For this review, take the finished solid that the model builds, in its own axes (mm). Face numbers are marked on the shaded views. A direction names the side the tool comes from. Round coordinates to 2 decimals unless told otherwise and drop trailing zeros. Order: outer loops, then holes, each group sorted by start corner. A loop starts at its lowest first (then second) coordinate and runs counter-clockwise, first axis right, second up.
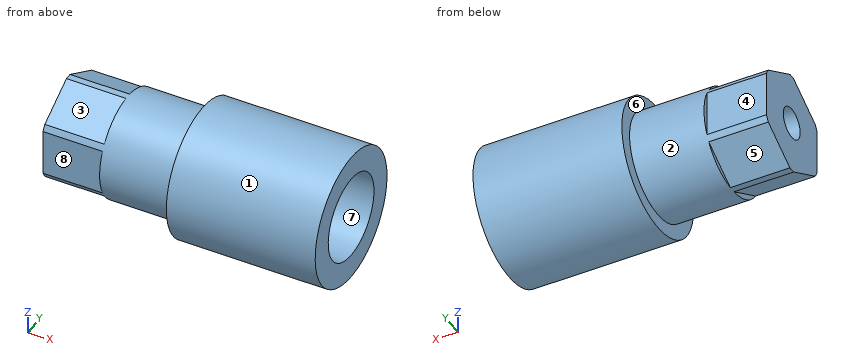
from build123d import *

# Parameters (mm, degrees)
CUT_EXTRUDE2_DEPTH = 12


with BuildPart() as part:
    # Sketch1 → Revolve1 (revolve)
    with BuildSketch(Plane.XY, mode=Mode.PRIVATE) as revolve1_sk:
        Polygon((57, -13.5), (27, -13.5), (27, -10.6), (0, -10.6), (0, -3.175), (34, -3.175), (34, -8.6), (57, -8.6), align=None)
    revolve(revolve1_sk.sketch.rotate(Axis((0, 0, 0), (1, 0, 0)), 270), axis=Axis((0, 0, 0), (1, 0, 0)))

    # Sketch2 → Cut-Extrude2 (cut)
    with BuildSketch(Plane.ZY):
        with BuildLine():
            Line((-10.578304925, 0.677838412), (-5.876177747, 8.822161588))
            ThreePointArc((-5.876177747, 8.822161588), (-9.17986928, 5.3), (-10.578304925, 0.677838412))
        make_face()
        with BuildLine():
            ThreePointArc((4.702127178, 9.5), (0, 10.6), (-4.702127178, 9.5))
            Line((-4.702127178, 9.5), (4.702127178, 9.5))
        make_face()
        with BuildLine():
            Line((-5.876177747, -8.822161588), (-10.578304925, -0.677838412))
            ThreePointArc((-10.578304925, -0.677838412), (-9.17986928, -5.3), (-5.876177747, -8.822161588))
        make_face()
        with BuildLine():
            ThreePointArc((10.578304925, 0.677838412), (9.17986928, 5.3), (5.876177747, 8.822161588))
            Line((5.876177747, 8.822161588), (10.578304925, 0.677838412))
        make_face()
        with BuildLine():
            Line((4.702127178, -9.5), (-4.702127178, -9.5))
            ThreePointArc((-4.702127178, -9.5), (0, -10.6), (4.702127178, -9.5))
        make_face()
        with BuildLine():
            ThreePointArc((5.876177747, -8.822161588), (9.17986928, -5.3), (10.578304925, -0.677838412))
            Line((10.578304925, -0.677838412), (5.876177747, -8.822161588))
        make_face()
    extrude(amount=-CUT_EXTRUDE2_DEPTH, mode=Mode.SUBTRACT)


solid = part.part
(1) Add section C-C on x = 5. Give the boundary of the cut face in (y, z) (3 decimals), plus the area to 3 significant figures.
(2) Tool access review of the marked faces 1, 2, 3 and 4: name each direction out of +Z, -Z, +X, -X, +Y, -Y from which nothing blocks a thin tool from reaching the whole face with its end or side.
(3) Wall thickness on L1, parallel to Y at x = 51, z = 0; L2, parallel to X at y = -6.75, z = 8.25; L3, parallel to X at y = 0.5, z = -7.5: over which ranges is each line inside the solid? List them lowest first.
(4) Add section A-A on z = 0. Give the boundary of the cut face in (x, y) (3 decimals), plus the area to 4 significant figures.
(5) Draft analysis for pull direction Y (two halves, no side actions). For the marked faces 5, 6, 7 and 8, state which applies: pulls with the +Y half, pulls with the -Y half, needs draft (parallel to the pull), parting line crosses it, or undercut.
(6) Clearance check with flat-ended pins moving along their axes: P1, Ø1, axis at x = 14, z = -8, coming from the +Y side; P2, Ø10, axis at y = 0.5, z = -0.5, coming from the +X side; P3, Ø4, axis at x = 9.5, y = 1.5, coming from the +Z side. State where each tip first meets the part, or that it passes through.
(7) Add section D-D on y = -6.75. Give the boundary of the cut face in (x, z).
(8) Add section B-B on y = 0. Give the boundary of the cut face in (x, z) (3 decimals), plus the area to 3 significant figures.
Here are the results:
1. outline: (-9.5, -4.702) arc R10.6 ccw to (-8.822, -5.876) - (-0.678, -10.578) arc R10.6 ccw to (0.678, -10.578) - (8.822, -5.876) arc R10.6 ccw to (9.5, -4.702) - (9.5, 4.702) arc R10.6 ccw to (8.822, 5.876) - (0.678, 10.578) arc R10.6 ccw to (-0.678, 10.578) - (-8.822, 5.876) arc R10.6 ccw to (-9.5, 4.702) - close; hole circle Ø6.35 at (0, 0)
1. area: 279 mm2
2. face 1: +X, -X
2. face 2: -X
2. face 3: +Z, -X, -Y
2. face 4: +Z, -Z, -X, +Y
3. L1: y = -13.5 to -8.6, 8.6 to 13.5
3. L2: x = 27 to 57
3. L3: x = 0 to 34
4. outline: (0, -9.5) - (12, -9.5) - (12, -10.6) - (27, -10.6) - (27, -13.5) - (57, -13.5) - (57, -8.6) - (34, -8.6) - (34, -3.175) - (0, -3.175) - close; (0, 3.175) - (34, 3.175) - (34, 8.6) - (57, 8.6) - (57, 13.5) - (27, 13.5) - (27, 10.6) - (12, 10.6) - (12, 9.5) - (0, 9.5) - close
4. area: 744.5 mm2
5. face 5: pulls with the +Y half
5. face 6: needs draft
5. face 7: undercut
5. face 8: pulls with the -Y half
6. P1: stops at y = 7.49
6. P2: stops at x = 34
6. P3: stops at z = 10.6
7. outline: (0, -7.07) - (12, -7.07) - (12, -8.17) - (27, -8.17) - (27, -11.69) - (57, -11.69) - (57, -5.33) - (34, -5.33) - (34, 5.33) - (57, 5.33) - (57, 11.69) - (27, 11.69) - (27, 8.17) - (12, 8.17) - (12, 7.07) - (0, 7.07) - close
8. outline: (0, -10.6) - (27, -10.6) - (27, -13.5) - (57, -13.5) - (57, -8.6) - (34, -8.6) - (34, -3.175) - (0, -3.175) - close; (0, 3.175) - (34, 3.175) - (34, 8.6) - (57, 8.6) - (57, 13.5) - (27, 13.5) - (27, 10.6) - (0, 10.6) - close
8. area: 771 mm2
